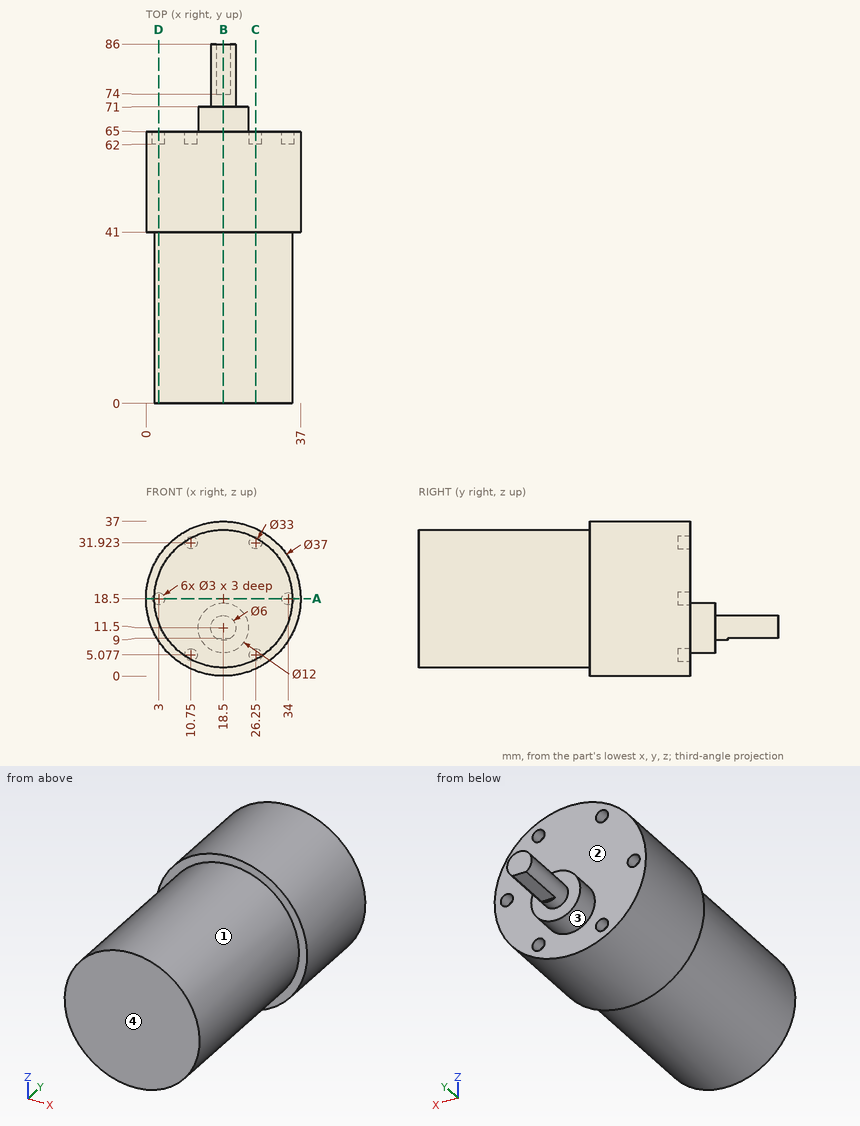
Geometry: see drawing. Coordinates: mm, zero at the bounding-box minimum. A direction names the side the tool comes from. Give positions to 0.01 mm unless a question says otherwise; leave off trailing zeros. Loops run counter-clockwise (first coordinate to the right, second up) from the corner with the lowest first, then second, coordinate; pieces in that order, holes last. Notation, with made-up numbers: (34, 57.25) - (78, 57.25) arc R12 ccw to (78, 77.25) - close; hole circle Ø4 at (-29, -11.5). An arc over 180 degrees is marked (long way). One line per question, with ' | ' between items. Start each with the question number.
(1) Section query D-D on x = 3. Return loops of the section in (y, z).
(2) Ray query, line 1 (X direction, y = 63.6, z = 18.5); line 2 (Z direction, x = 26, y = 63) (1 decimal); line 3 (Z direction, x = 18, y = 43). Return the intervals inside material, ascending. Write a range as from..to.
(3) Pull-direction query (X, two-part tool) for the marked faces 1 and 2; classes: released by +X, released by -X, zero draft, split by the parting line, or undercut.
(4) Contact query for flat-ended pins moving along their axis: pin 1 (8 mm diameter, centred on x = 18.5, y = 9, fed in from +Z); pin 2 (12 mm diameter, centred on x = 26, y = 62.5, fed in from +Z); pin 3 (1.5 mm diameter, centred on x = 11.5, z = 31.5, fed in from +Y); pin 4 (2 mm diameter, centred on y = 73, z = 5, fed in from +X). Output: stop coordinate, or through.
(5) Section query B-B on x = 18.5. Return loops of the section in (y, z), then the cut area to 3 significant figures.
(6) Reachability of the marked faces 3 and 4 from +Z, -Z, +X, -X, +Y, -Y: full face, straight path, thin tool, end or side. Return the list, or none.
(7) Section query A-A on z = 18.5. Return loops of the section in (x, y).
(8) Section query C-C on x = 26.25. Return loops of the section in (y, z).
The answers:
1) outline: (0, 12.84) - (41, 12.84) - (41, 8.4) - (65, 8.4) - (65, 17) - (62, 17) - (62, 20) - (65, 20) - (65, 28.6) - (41, 28.6) - (41, 24.16) - (0, 24.16) - close
2) line 1: 0..1.5, 4.5..32.5, 35.5..37 | line 2: 1.6..3.6, 6.6..30.4, 33.4..35.4 | line 3: 0.01..36.99
3) face 1: split by the parting line | face 2: zero draft
4) pin 1: z = 35 | pin 2: z = 36.94 | pin 3: y = 65 | pin 4: through
5) outline: (0, 2) - (41, 2) - (41, 0) - (65, 0) - (65, 5.5) - (71, 5.5) - (71, 8.5) - (74, 8.5) - (74, 9) - (86, 9) - (86, 14.5) - (71, 14.5) - (71, 17.5) - (65, 17.5) - (65, 37) - (41, 37) - (41, 35) - (0, 35) - close | area: 2,400 mm2
6) face 3: +Y | face 4: +Z, -Z, +X, -X, -Y
7) outline: (0, 41) - (2, 41) - (2, 0) - (35, 0) - (35, 41) - (37, 41) - (37, 65) - (35.5, 65) - (35.5, 62) - (32.5, 62) - (32.5, 65) - (4.5, 65) - (4.5, 62) - (1.5, 62) - (1.5, 65) - (0, 65) - close
8) outline: (0, 3.93) - (41, 3.93) - (41, 1.7) - (65, 1.7) - (65, 3.58) - (62, 3.58) - (62, 6.58) - (65, 6.58) - (65, 30.42) - (62, 30.42) - (62, 33.42) - (65, 33.42) - (65, 35.3) - (41, 35.3) - (41, 33.07) - (0, 33.07) - close
